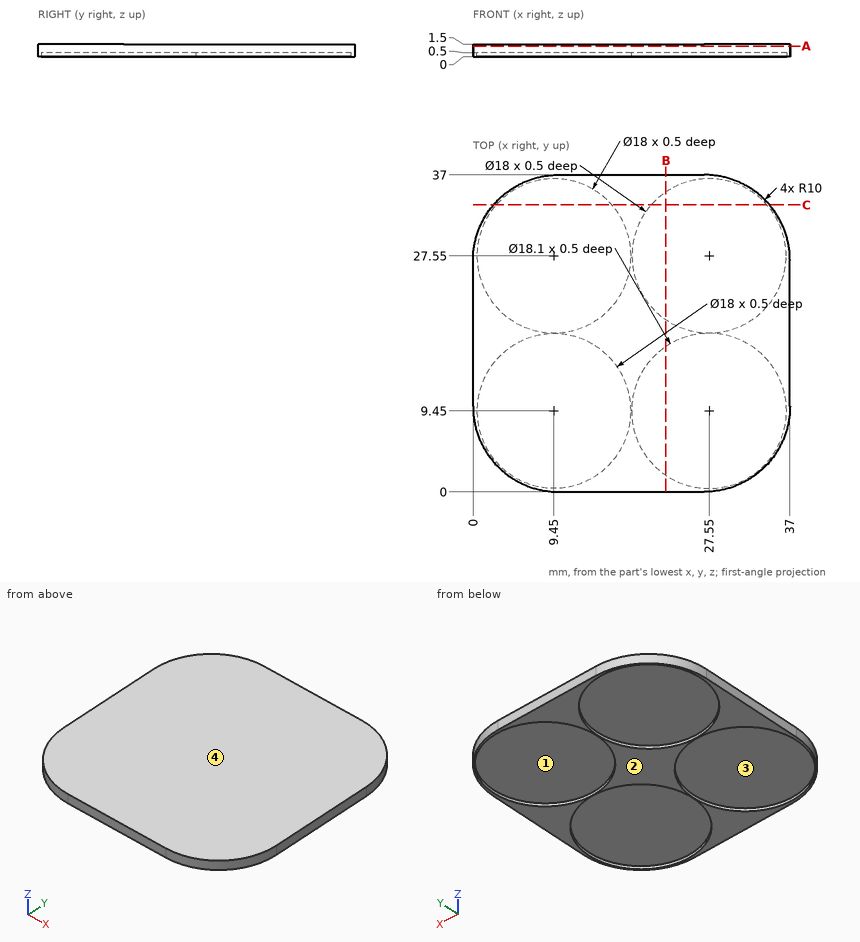
Verification items for this drawing (mm, ordinates from the low corner). A direction names the side the tool comes from. Give positions to 0.01 mm unless a question says otherwise; leave off trailing zeros. Loops run counter-clockwise (first coordinate to the right, second up) from the corner with the lowest first, then second, coordinate; pieces in that order, holes last. Notation, with made-up numbers: M 85,-22 L 143,-22 A20 cw 143,-8 Z; hole C -27,38 d8. An arc over 180 degrees is marked long. Write item = value, one per line. Start each with the question number.
1. Tool access check on the marked faces 3 and 4. Record the directions out of +Z, -Z, +X, -X, +Y, -Y that give a thin tool (end or side, any length) a straight path to the whole face; none if there is none.
2. Go/stop test with a flat-tipped pin: P1, Ø2, axis at x = 16.5, y = 6.5, coming from the -Z side. Record where the tip stops, or that it passes through.
3. Section check A-A, the plane z = 1.25. Enter the section's corners in (x, y), plus the area to 3 significant figures.
4. Section check C-C, the plane y = 33.5. Enter the section's corners in (x, z), plus the area to 3 significant figures.
5. Section check B-B, the plane x = 22.5. Enter the section's corners in (y, z).
6. Thickness scan on probe 1 along Y at (x, z) = (17, 0.3); probe 2 along X at (y, z) = (33, 0.1); probe 3 along X at (y, z) = (30, 0.1). Record the ranges inside material, lowest first.
7. Draft check along X on the marked faces 1 and 2. Enter one of: +X half, -X half, draft (parallel to the pull), parting line (faces both ways), or undercut.
Values follow:
q1.face_3 = -Z
q1.face_4 = +Z, +X, -X, +Y, -Y
q2.P1 = 0.5
q3.outline = M 0,10 A10 ccw 10,0 L 27,0 A10 ccw 37,10 L 37,27 A10 ccw 27,37 L 10,37 A10 ccw 0,27 Z
q3.area = 1,280 mm^2
q4.outline = M 2.4,0 L 2.7,0 L 2.7,0.5 L 16.2,0.5 L 16.2,0 L 20.8,0 L 20.8,0.5 L 34.3,0.5 L 34.3,0 L 34.6,0 L 34.6,1.5 L 2.4,1.5 Z
q4.area = 34.8 mm^2
q5.outline = M 0,0 L 1.94,0 L 1.94,0.5 L 16.96,0.5 L 16.96,0 L 20.1,0 L 20.1,0.5 L 35,0.5 L 35,0 L 37,0 L 37,1.5 L 0,1.5 Z
q6.probe_1 = 0 to 4.55, 14.35 to 22.65, 32.45 to 37
q6.probe_2 = 2 to 2.29, 16.61 to 20.39, 34.71 to 35
q6.probe_3 = 0.46 to 0.79, 18.11 to 18.89, 36.21 to 36.54
q7.face_1 = undercut
q7.face_2 = draft
